from build123d import *

# Parameters (mm, degrees)
F0_R     = 8.249045
F1_DEPTH = 32.5


with BuildPart() as f1:
    # F0 (on Right) → F1 (new body)
    with BuildSketch(Plane.YZ):
        Polygon((38.824608, 0.172873), (19.262591, 33.709534), (-19.562017, 33.53666), (-38.824608, -0.172873), (-19.262591, -33.709534), (19.562017, -33.53666), align=None)
        with Locations((0, -20.395683)):
            Circle(F0_R, mode=Mode.SUBTRACT)
    extrude(amount=F1_DEPTH)


solid = f1.part
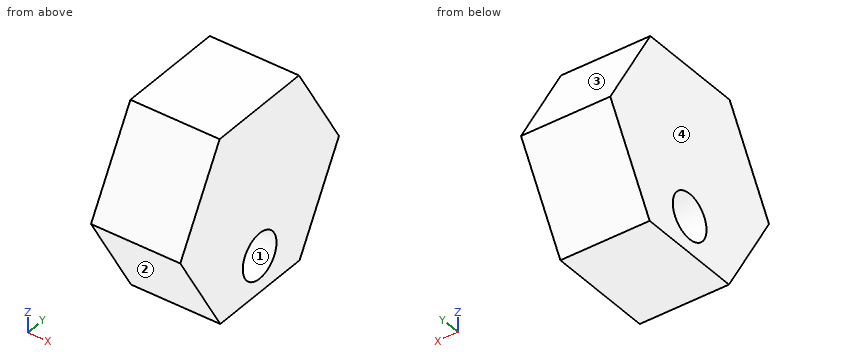
Design review of the part built by this model. Coordinates are the model's own, in mm. Face numbers are marked on the shaded views. Give positions to 0.01 mm unless a question says otherwise; leave off trailing zeros. Loops run counter-clockwise (first coordinate to the right, second up) from the corner with the lowest first, then second, coordinate; pieces in that order, holes last. Notation, with made-up numbers: M 8.25,11 L 19.25,11 A23 cw 19.25,23 Z; hole C 89.5,47.5 d11. An arc over 180 degrees is marked long. Write item = value, one per line.
Q1. Insertion check: pin 1 (5 mm diameter, centred on x = 11.5, y = 19.5, fed in from +Z); pin 2 (10 mm diameter, centred on y = 0, z = -20.4, fed in from -X); pin 3 (5 mm diameter, centred on x = 11.5, y = -12, fed in from +Z); pin 4 (6 mm diameter, centred on x = 12, z = -4, fed in from -Y). Each pin has a flat end and moves straight along its axis. Give the tip position at first contact, or say it passes through.
Output values:
pin_1 = 33.71
pin_2 = through
pin_3 = 33.58
pin_4 = -38.34
Q2. We need section A-A (y = 5). Give the boundary of the cut face in (x, z), plus the area to 3 significant figures.
Output values:
outline = M 0,-33.6 L 32.5,-33.6 L 32.5,-26.96 L 0,-26.96 Z; M 0,-13.83 L 32.5,-13.83 L 32.5,33.65 L 0,33.65 Z
area = 1,760 mm^2
Q3. Draft analysis for pull direction Y (two halves, no side actions). For the marked faces 1, 2, 3 and 4, state which applies: +Y half, -Y half, draft (parallel to the pull), parting line (faces both ways), or undercut.
Output values:
face_1 = undercut
face_2 = -Y half
face_3 = +Y half
face_4 = draft
Q4. We need section B-B (x = 21). Give the boundary of the cut face in (y, z).
Output values:
outline = M -38.82,-0.17 L -19.26,-33.71 L 19.56,-33.54 L 38.82,0.17 L 19.26,33.71 L -19.56,33.54 Z; hole C 0,-20.4 d16.5
Q5. We need section C-C (z = -14). Give the boundary of the cut face in (x, y).
Output values:
outline = M 0,-30.76 L 32.5,-30.76 L 32.5,-5.21 L 0,-5.21 Z; M 0,5.21 L 32.5,5.21 L 32.5,30.73 L 0,30.73 Z
Q6. To check wall thickness, follow line 1 (Z direction, x = 30, y = -16) (3 decimals); line 2 (Z direction, x = 18.5, y = 0); line 3 (Z direction, x = 29, y = 1). State the ranges of each line that lie inside material, in increasing order. Write a range as [from, to].
Output values:
line_1 = [-33.695, 33.553]
line_2 = [-33.62, -28.64], [-12.15, 33.62]
line_3 = [-33.62, -28.58], [-12.21, 33.63]
Q7. We need section D-D (y = 21.5). Give the boundary of the cut face in (x, z), plus the area to 3 significant figures.
Output values:
outline = M 0,-30.15 L 32.5,-30.15 L 32.5,29.87 L 0,29.87 Z
area = 1,950 mm^2
